Geometry: final body of the model. Coordinates: model frame, mm. Give positions to 0.01 mm unless a question says otherwise; leave off trailing zeros. Loops run counter-clockwise (first coordinate to the right, second up) from the corner with the lowest first, then second, coordinate; pieces in that order, holes last. Notation, with made-up numbers: (-30, 67) -> (18, 67) arc R29 cw to (18, 102) -> close; hole circle Ø5 at (79, 47.25). An arc over 180 degrees is marked (long way). Answer in a Markdown table with one row per item. Add a question column.
from build123d import *

# Parameters (mm, degrees)
F1_W      = 29.21
F1_H      = 29.21
F2_DEPTH  = 831.85
F3_W      = 29.21
F3_H      = 29.21
F4_DEPTH  = 685.8
F7_DEPTH  = 38.1
F10_DEPTH = 38.1


with BuildPart() as f2:
    # F1 (on Front) → F2 (new body, symmetric)
    with BuildSketch(Plane.XZ):
        with BuildLine():
            ThreePointArc((-685.8, 15.24), (-686.915923, 17.934077), (-689.61, 19.05))
            Line((-689.61, 19.05), (-720.09, 19.05))
            ThreePointArc((-720.09, 19.05), (-722.784077, 17.934077), (-723.9, 15.24))
            Line((-723.9, 15.24), (-723.9, -15.24))
            ThreePointArc((-723.9, -15.24), (-722.784077, -17.934077), (-720.09, -19.05))
            Line((-720.09, -19.05), (-689.61, -19.05))
            ThreePointArc((-689.61, -19.05), (-686.915923, -17.934077), (-685.8, -15.24))
            Line((-685.8, -15.24), (-685.8, 15.24))
        make_face()
        with Locations((-704.85, 0)):
            Rectangle(F1_W, F1_H, mode=Mode.SUBTRACT)
        with BuildLine():
            ThreePointArc((723.9, 15.24), (722.784077, 17.934077), (720.09, 19.05))
            Line((720.09, 19.05), (689.61, 19.05))
            ThreePointArc((689.61, 19.05), (686.915923, 17.934077), (685.8, 15.24))
            Line((685.8, 15.24), (685.8, -15.24))
            ThreePointArc((685.8, -15.24), (686.915923, -17.934077), (689.61, -19.05))
            Line((689.61, -19.05), (720.09, -19.05))
            ThreePointArc((720.09, -19.05), (722.784077, -17.934077), (723.9, -15.24))
            Line((723.9, -15.24), (723.9, 15.24))
        make_face()
        with Locations((704.85, 0)):
            Rectangle(F1_W, F1_H, mode=Mode.SUBTRACT)
    extrude(amount=F2_DEPTH, both=True)

    # F3 (on Right) → F4 (join, symmetric)
    with BuildSketch(Plane.YZ):
        with BuildLine():
            ThreePointArc((-793.75, 15.24), (-794.865923, 17.934077), (-797.56, 19.05))
            Line((-797.56, 19.05), (-828.04, 19.05))
            ThreePointArc((-828.04, 19.05), (-830.734077, 17.934077), (-831.85, 15.24))
            Line((-831.85, 15.24), (-831.85, -15.24))
            ThreePointArc((-831.85, -15.24), (-830.734077, -17.934077), (-828.04, -19.05))
            Line((-828.04, -19.05), (-797.56, -19.05))
            ThreePointArc((-797.56, -19.05), (-794.865923, -17.934077), (-793.75, -15.24))
            Line((-793.75, -15.24), (-793.75, 15.24))
        make_face()
        with Locations((-812.8, 0)):
            Rectangle(F3_W, F3_H, mode=Mode.SUBTRACT)
        with BuildLine():
            ThreePointArc((831.85, 15.24), (830.734077, 17.934077), (828.04, 19.05))
            Line((828.04, 19.05), (797.56, 19.05))
            ThreePointArc((797.56, 19.05), (794.865923, 17.934077), (793.75, 15.24))
            Line((793.75, 15.24), (793.75, -15.24))
            ThreePointArc((793.75, -15.24), (794.865923, -17.934077), (797.56, -19.05))
            Line((797.56, -19.05), (828.04, -19.05))
            ThreePointArc((828.04, -19.05), (830.734077, -17.934077), (831.85, -15.24))
            Line((831.85, -15.24), (831.85, 15.24))
        make_face()
        with Locations((812.8, 0)):
            Rectangle(F3_W, F3_H, mode=Mode.SUBTRACT)
    extrude(amount=F4_DEPTH, both=True)

    # F6 (on offset) → F7 (join)
    with BuildSketch(Plane.XZ.offset(831.85)):
        Polygon((-685.8, 15.24), (-685.8, 19.05), (-689.61, 19.05), align=None)
        Polygon((685.8, 15.24), (689.61, 19.05), (685.8, 19.05), align=None)
        Polygon((-689.61, -19.05), (-685.8, -19.05), (-685.8, -15.24), align=None)
        Polygon((685.8, -15.24), (685.8, -19.05), (689.61, -19.05), align=None)
    extrude(amount=-F7_DEPTH)

    # F9 (on offset) → F10 (join)
    with BuildSketch(Plane(origin=(0, 831.85, 0), x_dir=(1, 0, 0), z_dir=(0, 1, 0))):
        Polygon((-685.8, 15.24), (-685.8, 19.05), (-689.61, 19.05), align=None)
        Polygon((689.61, 19.05), (685.8, 19.05), (685.8, 15.24), align=None)
        Polygon((685.8, -15.24), (685.8, -19.05), (689.61, -19.05), align=None)
        Polygon((-689.61, -19.05), (-685.8, -19.05), (-685.8, -15.24), align=None)
    extrude(amount=-F10_DEPTH)


solid = f2.part
(1) Cut plane B-B on x = 164.5. Return the cut outline in (y, z) (3 decimals).
(2) Cut plane A-A on z = 3. Return the cut outline in (x, y) (3 decimals), then the cut area to 3 significant figures.
(3) Cut plane C-C on y = 648. Return the cut outline in (x, z) (3 decimals), then the cut area to 3 significant figures.
(4) Material intervals for line 1 along Y through (x, z) = (-370, 5) (3 decimals); line 2 along X through (y, z) = (-331, 9) (3 decimals); line 3 along Y through (x, z) = (105.5, -15), sorted ascending. Write a range as from..to.
(5) Pin query (flat end, axial travel): pin 1 Ø1.1 at (y, z) = (-795.5, -18) entering from +X; pin 2 Ø1.1 at (y, z) = (830.5, -17.5) entering from -X; pin 3 Ø1.1 at (y, z) = (-794.5, 17) entering from -X. Return the tip coordinate at first contact, or that it passes through.
Answer list:
| question | item | result |
|---|---|---|
| 1 | outline | (-831.85, -15.24) arc R3.81 ccw to (-828.04, -19.05) -> (-797.56, -19.05) arc R3.81 ccw to (-793.75, -15.24) -> (-793.75, 15.24) arc R3.81 ccw to (-797.56, 19.05) -> (-828.04, 19.05) arc R3.81 ccw to (-831.85, 15.24) -> close; (793.75, -15.24) arc R3.81 ccw to (797.56, -19.05) -> (828.04, -19.05) arc R3.81 ccw to (831.85, -15.24) -> (831.85, 15.24) arc R3.81 ccw to (828.04, 19.05) -> (797.56, 19.05) arc R3.81 ccw to (793.75, 15.24) -> close; hole (-827.405, -14.605) -> (-798.195, -14.605) -> (-798.195, 14.605) -> (-827.405, 14.605) -> close; hole (798.195, -14.605) -> (827.405, -14.605) -> (827.405, 14.605) -> (798.195, 14.605) -> close |
| 2 | outline | (-723.9, -831.85) -> (-719.455, -831.85) -> (-719.455, 831.85) -> (-723.9, 831.85) -> close; (-690.245, -831.85) -> (690.245, -831.85) -> (690.245, 831.85) -> (-690.245, 831.85) -> close; (719.455, -831.85) -> (723.9, -831.85) -> (723.9, 831.85) -> (719.455, 831.85) -> close; hole (-685.8, -827.405) -> (685.8, -827.405) -> (685.8, -798.195) -> (-685.8, -798.195) -> close; hole (-685.8, -793.75) -> (685.8, -793.75) -> (685.8, 793.75) -> (-685.8, 793.75) -> close; hole (-685.8, 798.195) -> (685.8, 798.195) -> (685.8, 827.405) -> (-685.8, 827.405) -> close |
| 2 | area | 54,000 mm² |
| 3 | outline | (-723.9, -15.24) arc R3.81 ccw to (-720.09, -19.05) -> (-689.61, -19.05) arc R3.81 ccw to (-685.8, -15.24) -> (-685.8, 15.24) arc R3.81 ccw to (-689.61, 19.05) -> (-720.09, 19.05) arc R3.81 ccw to (-723.9, 15.24) -> close; (685.8, -15.24) arc R3.81 ccw to (689.61, -19.05) -> (720.09, -19.05) arc R3.81 ccw to (723.9, -15.24) -> (723.9, 15.24) arc R3.81 ccw to (720.09, 19.05) -> (689.61, 19.05) arc R3.81 ccw to (685.8, 15.24) -> close; hole (-719.455, -14.605) -> (-690.245, -14.605) -> (-690.245, 14.605) -> (-719.455, 14.605) -> close; hole (690.245, -14.605) -> (719.455, -14.605) -> (719.455, 14.605) -> (690.245, 14.605) -> close |
| 3 | area | 1,170 mm² |
| 4 | line 1 | y = -831.85..-827.405, -798.195..-793.75, 793.75..798.195, 827.405..831.85 |
| 4 | line 2 | x = -723.9..-719.455, -690.245..-685.8, 685.8..690.245, 719.455..723.9 |
| 4 | line 3 | y = -831.85..-793.75, 793.75..831.85 |
| 5 | pin 1 | stops at x = 723.19 |
| 5 | pin 2 | stops at x = -723.49 |
| 5 | pin 3 | stops at x = -723.7 |
